Answer from the drawing. Dimensions are ordinates in mm from the lowest x, y and z of the part. A direction names the side the tool comes from. Coordinates: 2 decimals unless noted, no trailing zeros. Write each loop counter-clockwise with the first axis right and the second up, starting at its lowest first coordinate (ties: lowest second). Pieces come first, ordered by that corner, then holes. Notation, with made-up numbers: (-1, 38) - (48, 38) arc R25 cw to (48, 52) - close; hole circle Ø3 at (-25, -2). An arc over 180 degrees is marked (long way). Use one line per item in the form item = value. Start each with the question number.
Item 1: A cutting plane is placed at B-B (z = 22.5). Write down the section's boundary in (x, y), then the cut area to 3 significant figures.
Item 2: Given pin 1 (2 mm diameter, centred on x = 6.35, z = 36.4, fed in from +Y); pin 2 (8 mm diameter, centred on x = 19, z = 9, fed in from -Y); pin 3 (7 mm diameter, centred on x = 82.55, z = 14.4, fed in from -Y), each flat-ended and moving along its own axis, determine where each tip first touches the part or whether it passes through.
Item 3: Consider probe 1 along Z at (x, y) = (19.05, 11.25) (1 decimal); probe 2 along Z at (x, y) = (6.35, 10) (1 decimal); probe 3 along Y at (x, z) = (15.5, 34). Determine where each line is inside the solid, lowest interval first.
Item 4: For the marked faces 1, 2 and 3, determine the directions among +Z, -Z, +X, -X, +Y, -Y from which every point of the face is accessible in a straight line to the end or side of a thin tool.
Item 5: A cutting plane is placed at D-D (y = 8.5). Give the number of separate pieces and of enclosed holes in the cut face, then the cut area to 3 significant figures.
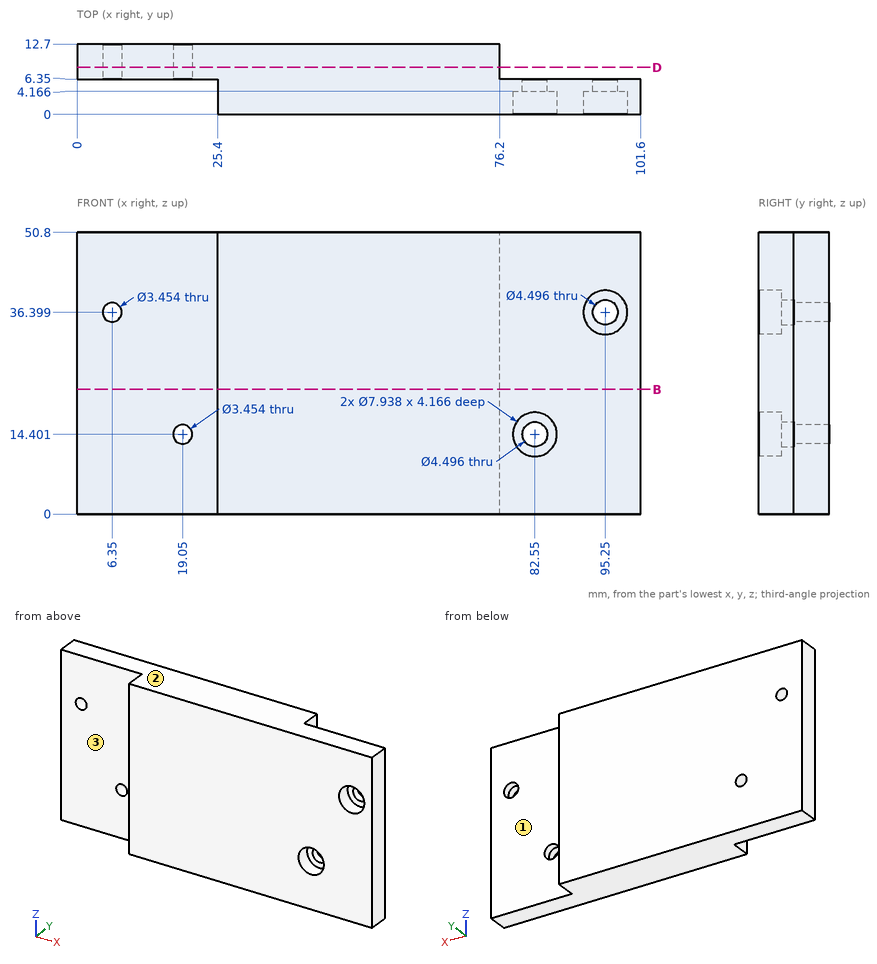
Answer:
q1.outline = (0, 6.35) - (25.4, 6.35) - (25.4, 0) - (101.6, 0) - (101.6, 6.35) - (76.2, 6.35) - (76.2, 12.7) - (0, 12.7) - close
q1.area = 968 mm²
q2.pin_1 = through
q2.pin_2 = 6.35
q2.pin_3 = 4.17
q3.probe_1 = 0 to 12.7, 16.1 to 50.8
q3.probe_2 = 0 to 34.7, 38.1 to 50.8
q3.probe_3 = 6.35 to 12.7
q4.face_1 = +Z, -Z, +X, +Y
q4.face_2 = +Z, +X, -X, +Y, -Y
q4.face_3 = +Z, -Z, -X, -Y
q5.separate_pieces = 1
q5.enclosed_holes = 2
q5.area = 3,850 mm²
